The drawing under review shows one solid part. Ordinate dimensions are in mm from its lowest x, y, z. Give positions to 0.01 mm unless a question says otherwise; leave off trailing zeros. Order: outer loops, then holes, each group sorted by start corner. A loop starts at its lowest first (then second) coordinate and runs counter-clockwise, first axis right, second up. Notation, with made-up numbers: (-1.75, -31) -> (12.25, -31) arc R26 cw to (12.25, -9) -> close; hole circle Ø7 at (49.5, 18). An arc over 180 degrees is marked (long way). One line per item, written item: value.
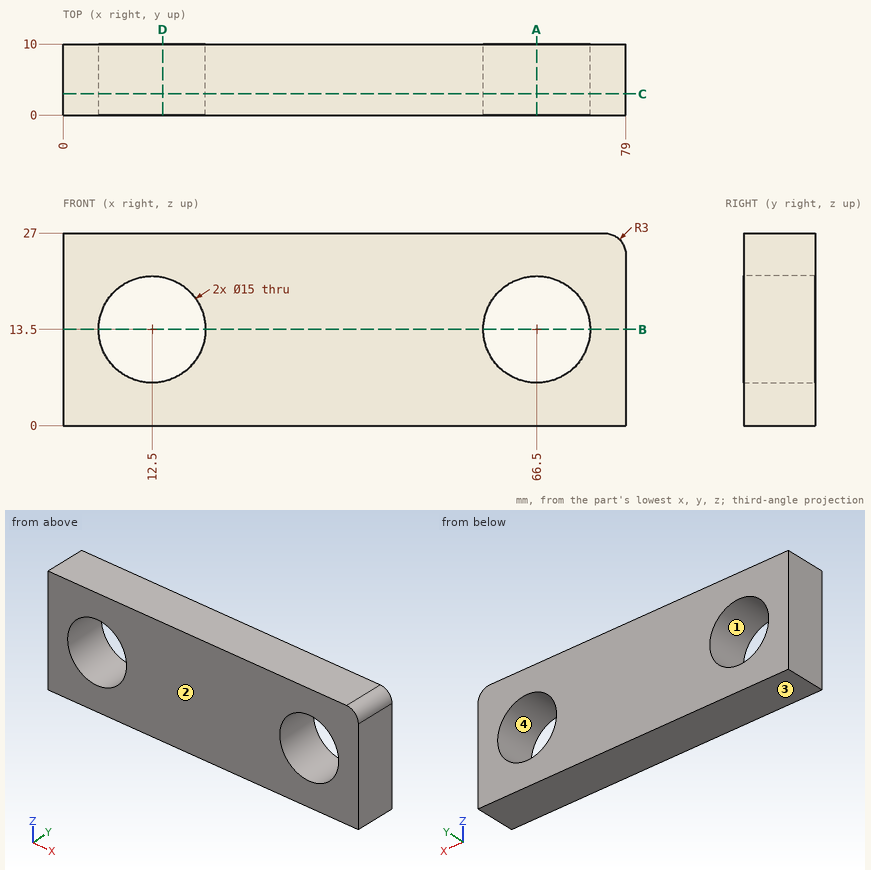
Item 1: Add section C-C on y = 3. Give the boundary of the cut face in (x, z).
Returned:
outline: (0, 0) -> (79, 0) -> (79, 24) arc R3 ccw to (76, 27) -> (0, 27) -> close; hole circle Ø15 at (12.5, 13.5); hole circle Ø15 at (66.5, 13.5)
Item 2: Add section B-B on z = 13.5. Give the boundary of the cut face in (x, y), plus the area to 3 significant figures.
Returned:
outline: (0, 0) -> (5, 0) -> (5, 10) -> (0, 10) -> close; (20, 0) -> (59, 0) -> (59, 10) -> (20, 10) -> close; (74, 0) -> (79, 0) -> (79, 10) -> (74, 10) -> close
area: 490 mm²
Item 3: Add section D-D on x = 14. Give the boundary of the cut face in (y, z).
Returned:
outline: (0, 0) -> (10, 0) -> (10, 6.15) -> (0, 6.15) -> close; (0, 20.85) -> (10, 20.85) -> (10, 27) -> (0, 27) -> close
Item 4: Draft analysis for pull direction Z (two halves, no side actions). For the marked faces 1, 2, 3 and 4, state which applies: pulls with the +Z half, pulls with the -Z half, needs draft (parallel to the pull), parting line crosses it, or undercut.
Returned:
face 1: undercut
face 2: needs draft
face 3: pulls with the -Z half
face 4: undercut
Item 5: To check wall thickness, follow line 1 along X through (y, z) = (8.25, 13.5); line 2 along X through (y, z) = (9, 7); line 3 along Z through (x, y) = (16.5, 3.25). State the ranges of each line that lie inside material, in increasing order. Write a range as from..to.
Returned:
line 1: 0..5, 20..59, 74..79
line 2: 0..8.76, 16.24..62.76, 70.24..79
line 3: 0..7.16, 19.84..27
Item 6: Add section A-A on x = 66.5. Give the boundary of the cut face in (y, z), plus the area to 3 significant figures.
Returned:
outline: (0, 0) -> (10, 0) -> (10, 6) -> (0, 6) -> close; (0, 21) -> (10, 21) -> (10, 27) -> (0, 27) -> close
area: 120 mm²
